Answer from the drawing. Dimensions are ordinates in mm from the lowest x, y and z of the part. A direction names the side the tool comes from. Round coordinates to 2 decimals unless told otherwise and drop trailing zeros. Loops run counter-clockwise (first coordinate to the right, second up) from the corner with the lowest first, then second, coordinate; pieces in that order, holes last. Notation, with made-up numbers: (52, -15) - (76, -15) arc R37 cw to (76, 21) - close; hole circle Ø4 at (63.25, 32). An arc over 180 degrees is marked (long way). Write item = value, one per line. Start each with the question number.
1) Given pin 1 Ø1.7 at (y, z) = (11, 75) entering from -X; pin 2 Ø1 at (y, z) = (9, 13) entering from -X; pin 3 Ø4 at (x, z) = (13, 45) entering from +Y, each flat-ended and moving along its own axis, determine where each tip first touches the part or whether it passes through.
2) Section D-D, the plane y = 10 is taken. Give the number of separate pieces and of enclosed holes in the cut face, and give its area (3 significant figures).
3) Section A-A, the plane z = 80 is taken. Determine the outline of the cut face in (x, y), and give its area (3 significant figures).
4) Straight lines are drawn through the part: line 1 along Z through (x, y) = (7.45, 10); line 2 along Y through (x, z) = (10, 2.2); line 3 along Y through (x, z) = (12.5, 80). For each, find the intervals that lie inside material, in ascending order.
5) Section C-C, the plane x = 17 is taken. Determine the outline of the cut face in (y, z).
6) Section B-B, the plane x = 10 is taken. Determine the outline of the cut face in (y, z), and give its area (3 significant figures).
7) A tool of negligible diameter and unlimited length cuts with its end or side. For the marked faces 1 and 2, from which of +Z, -Z, +X, -X, +Y, -Y can it reach the whole face along a straight path? Write none if from no direction.
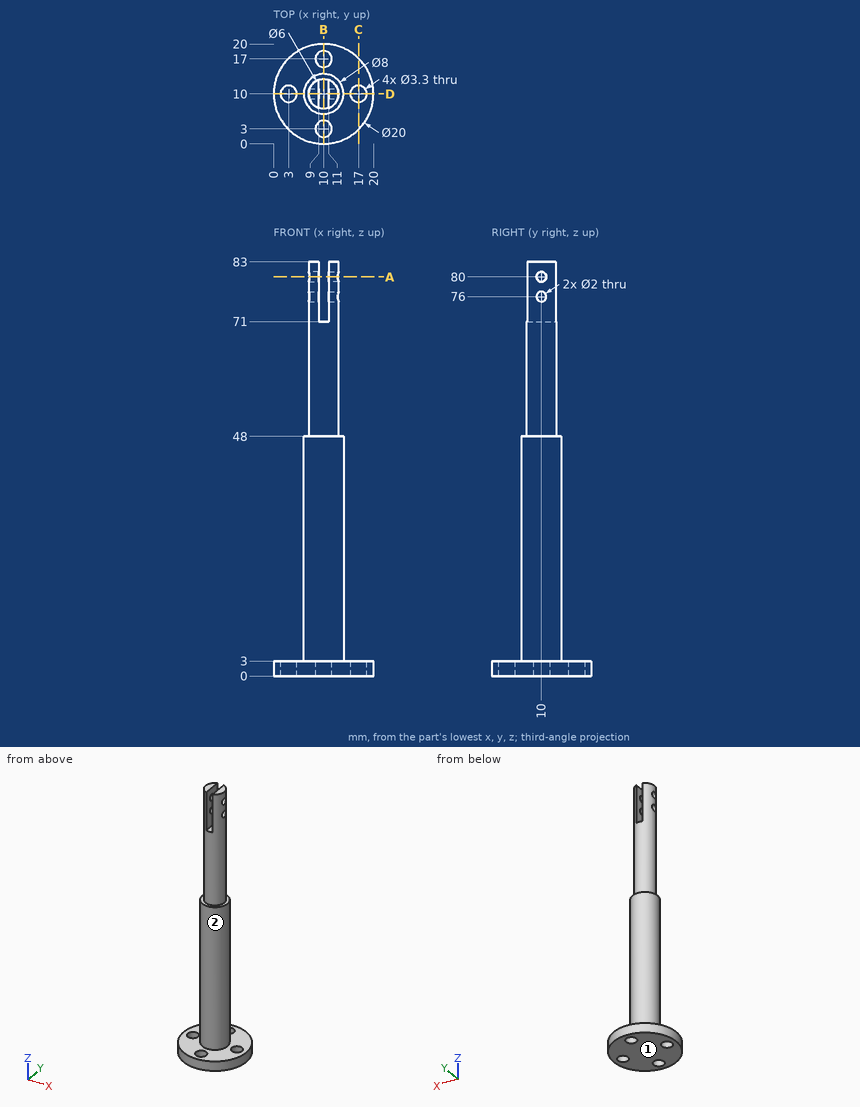
Geometry check:
q1.pin_1 = 7
q1.pin_2 = 6.03
q1.pin_3 = 13.87
q2.separate_pieces = 7
q2.enclosed_holes = 0
q2.area = 570 mm2
q3.outline = (7.17, 9) arc R3 ccw to (9, 7.17) - (9, 9) - close; (7.17, 11) - (9, 11) - (9, 12.83) arc R3 ccw to start; (11, 7.17) arc R3 ccw to (12.83, 9) - (11, 9) - close; (11, 11) - (12.83, 11) arc R3 ccw to (11, 12.83) - close
q3.area = 8.73 mm2
q4.line_1 = 0 to 75, 77 to 79, 81 to 83
q4.line_2 = 0 to 1.35, 4.65 to 15.35, 18.65 to 20
q4.line_3 = 8.34 to 9, 11 to 11.66
q5.outline = (2.86, 0) - (8.35, 0) - (8.35, 3) - (2.86, 3) - close; (11.65, 0) - (17.14, 0) - (17.14, 3) - (11.65, 3) - close
q6.outline = (0, 0) - (1.35, 0) - (1.35, 3) - (0, 3) - close; (4.65, 0) - (15.35, 0) - (15.35, 3) - (14, 3) - (14, 48) - (13, 48) - (13, 71) - (7, 71) - (7, 48) - (6, 48) - (6, 3) - (4.65, 3) - close; (18.65, 0) - (20, 0) - (20, 3) - (18.65, 3) - close
q6.area = 538 mm2
q7.face_1 = -Z, +X, -X, +Y, -Y
q7.face_2 = +Z
